```python
from build123d import *

# Parameters (mm, degrees)
SKETCH1_R                = 3.75
BOSS_EXTRUDE1_DEPTH      = 25
BOSS_EXTRUDE10_START     = -1e-07
BOSS_EXTRUDE10_OUTLINE_R = 3.75
BOSS_EXTRUDE10_DEPTH     = 53.7500002
BOSS_EXTRUDE10_START_2   = -5
BOSS_EXTRUDE10_2_DEPTH   = 10
CUT_REVOLVE2_START       = -5
CUT_REVOLVE2_OUTLINE_W   = 10
CUT_REVOLVE2_OUTLINE_H   = 33.75
CUT_REVOLVE2_DEPTH       = 10
SKETCH10_R               = 3.75
BOSS_EXTRUDE18_DEPTH     = 50
SKETCH11_R               = 2.5
CUT_EXTRUDE12_DEPTH      = 50
CUT_EXTRUDE14_START      = -21.25
SKETCH13_R               = 2.5
CUT_EXTRUDE14_DEPTH      = 21.25


with BuildPart() as part:
    # Sketch1 → Boss-Extrude1 (new, symmetric)
    with BuildSketch(Plane.XY):
        Circle(SKETCH1_R)
    extrude(amount=BOSS_EXTRUDE1_DEPTH, both=True)

    # Boss-Extrude10: read off the stored shape, not the designer's step
    # Boss-Extrude10 outline → Boss-Extrude10 (add)
    with BuildSketch(Plane(origin=(0, 0, 0), x_dir=(1, 0, 0), z_dir=(0, 1, 0)).offset(BOSS_EXTRUDE10_START)):
        Circle(BOSS_EXTRUDE10_OUTLINE_R)
    extrude(amount=BOSS_EXTRUDE10_DEPTH)

    # Boss-Extrude10 2 outline → Boss-Extrude10 2 (cut)
    with BuildSketch(Plane.XY.offset(BOSS_EXTRUDE10_START_2)):
        with BuildLine():
            Line((-5, 50), (-3.75, 50))
            ThreePointArc((-3.75, 50), (-2.651650429, 52.651650429), (0, 53.75))
            Line((0, 53.75), (-5, 53.7500001))
            Line((-5, 53.7500001), (-5, 50))
        make_face()
        with BuildLine():
            Line((5, 53.7500001), (0, 53.75))
            ThreePointArc((0, 53.75), (2.651650429, 52.651650429), (3.75, 50))
            Line((3.75, 50), (5, 50))
            Line((5, 50), (5, 53.7500001))
        make_face()
    extrude(amount=BOSS_EXTRUDE10_2_DEPTH, mode=Mode.SUBTRACT)

    # Cut-Revolve2: read off the stored shape, not the designer's step
    # Cut-Revolve2 outline → Cut-Revolve2 (cut)
    with BuildSketch(Plane(origin=(0, 0, 0), x_dir=(0, 0, -1), z_dir=(1, 0, 0)).offset(CUT_REVOLVE2_START)):
        with Locations((0, 38.125)):
            Rectangle(CUT_REVOLVE2_OUTLINE_W, CUT_REVOLVE2_OUTLINE_H)
    extrude(amount=CUT_REVOLVE2_DEPTH, mode=Mode.SUBTRACT)

    # Sketch10 → Boss-Extrude18 (add)
    with BuildSketch(Plane(origin=(0, 0, 0), x_dir=(0, 0, -1), z_dir=(1, 0, 0))):
        Circle(SKETCH10_R)
    extrude(amount=BOSS_EXTRUDE18_DEPTH)

    # Sketch11 → Cut-Extrude12 (cut)
    with BuildSketch(Plane(origin=(0, 0, -25), x_dir=(-1, 0, 0), z_dir=(0, 0, -1))):
        with Locations(Location((0, 0, 0), (0, 0, 180))):
            Circle(SKETCH11_R)
    extrude(amount=-CUT_EXTRUDE12_DEPTH, mode=Mode.SUBTRACT)

    # Sketch13 → Cut-Extrude14 (cut)
    with BuildSketch(Plane(origin=(0, 21.25, 0), x_dir=(1, 0, 0), z_dir=(0, 1, 0)).offset(CUT_EXTRUDE14_START)):
        with Locations(Location((0, 0, 0), (0, 0, 270))):
            Circle(SKETCH13_R)
    extrude(amount=CUT_EXTRUDE14_DEPTH, mode=Mode.SUBTRACT)


solid = part.part
```
The listing builds one solid part. Answer for the finished solid, in the listing's coordinates (mm). A direction names the side the tool comes from. Round coordinates to 2 decimals unless told otherwise and drop trailing zeros. Write each loop counter-clockwise with the first axis right and the second up, starting at its lowest first coordinate (ties: lowest second). Pieces come first, ordered by that corner, then holes. Notation, with made-up numbers: (60, -9.5) -> (107, -9.5) arc R30 ccw to (107, 22.5) -> close; hole circle Ø2 at (-4.5, -31.75). An arc over 180 degrees is marked (long way). Answer as a JSON object with one key per item and string values. Group by question number.
Q1. Determine the mould class of faces 3 (the face through (-0.33, -2.48, -0.35)), 4 (the face through (-2.976, -2.282, 0.35)), 5 (the face through (24.65, -3.66, 0.81)) for opening direction X: pulls with the +X half, pulls with the -X half, needs draft (parallel to the pull), parting line crosses it, or undercut.
Q2. Section C-C (z = -16) is taken. Write down the section's boundary in (x, y), plus the area to 3 significant figures.
Q3. Each of these flat-tipped pins is pushed along its axis until it touches: pin 1 Ø4 at (x, z) = (0, 0) entering from +Y; pin 2 Ø3 at (x, y) = (32.5, 0) entering from -Z; pin 3 Ø4 at (x, z) = (4.5, 7.5) entering from -Y. Where does it stop, or does it pass through?
Q4. Section A-A (z = 0) is taken. Write down the section's boundary in (x, y).
Q5. A straight line is drawn through the part: line 1 along Z through (x, y) = (0, 14.5). Find the intervals that lie inside material, in ascending order.
Q6. Which of the six approach directions +Z, -Z, +X, -X, +Y, -Y give full straight-line access (tool end or side, diameter ignored) to faces 1 (the face through (-3, 21.25, 0)), 2 (the face through (-3.746, 12.837, -0.165))?
Q7. Section B-B (y = 1.5) is taken. Write down the section's boundary in (x, z), plus the area to 3 significant figures.
Check values:
{
 "1": {"face 3": "undercut", "face 4": "parting line crosses it", "face 5": "needs draft"},
 "2": {"outline": "circle Ø7.5 at (0, 0); hole circle Ø5 at (0, 0)", "area": "24.5 mm^2"},
 "3": {"pin 1": "y = -1.5", "pin 2": "z = -3.75", "pin 3": "y = -2.8"},
 "4": {"outline": "(-3.75, 0) arc R3.75 ccw to (0, -3.75) -> (50, -3.75) -> (50, 3.75) -> (3.75, 3.75) -> (3.75, 21.25) -> (2.5, 21.25) -> (2.5, 0) arc R2.5 cw to (-2.5, 0) -> (-2.5, 21.25) -> (-3.75, 21.25) -> close"},
 "5": {"line 1": "-3.75 to -2.5, 2.5 to 3.75"},
 "6": {"face 1": "+Z, -Z, +X, -X, +Y", "face 2": "+Y"},
 "7": {"outline": "(-3.44, -25) -> (-2, -25) -> (-2, -1.5) arc R2.5 cw to (-2, 1.5) -> (-2, 25) -> (-3.44, 25) -> (-3.44, 1.5) arc R3.75 ccw to (-3.44, -1.5) -> close; (2, -25) -> (3.44, -25) -> (3.44, -3.44) -> (50, -3.44) -> (50, 3.44) -> (3.44, 3.44) -> (3.44, 25) -> (2, 25) -> (2, 1.5) arc R2.5 cw to (2, -1.5) -> close", "area": "462 mm^2"}
}
